The model under review builds one solid part; all positions refer to its coordinate system, in mm. Coordinates: 2 decimals unless noted, no trailing zeros. Loops run counter-clockwise (first coordinate to the right, second up) from the corner with the lowest first, then second, coordinate; pieces in that order, holes last. Notation, with made-up numbers: (76, 67.5) - (90, 67.5) arc R17 cw to (90, 96.5) - close; hole circle Ø5 at (75, 42). An arc over 180 degrees is marked (long way). Answer in a Markdown table with one row per item. Add a question column.
(1) We need section C-C on y = -3. Write out the cut boundary in (x, z).
(2) For P1, Ø4.5, axis at x = -5, y = 0, coming from the -Z side, flat-tipped, find the tip position at first contact; note if it passes through.
(3) We need section A-A on x = 15. Write out the cut boundary in (y, z).
(4) We need section B-B on z = 0.1. Give the number of separate pieces and of enclosed holes in the cut face, plus the area to 3 significant figures.
(5) For line 1 along Y through (x, z) = (-35, 0.25); line 2 along Y through (x, z) = (-26, 0.2); line 3 along X through (y, z) = (2.75, 0.2), list the stretches that pass through material, from the lowest coordinate up.
(6) Mouldability with a two-part tool opening along X and no side actions: class faces 1 (the flat face through (-1, 0, 0.5)), 2 (the cylindrical face through (-3.002, 0.088, 0.246)), 3 (the cylindrical face through (33.153, -0.766, 0.246)), 4 (the cylindrical face through (-50, -0.1, 0.2)) as +X half, -X half, draft (parallel to the pull), parting line (faces both ways), or undercut.
Autodesk Inventor part; units mm, degrees
ref_plane "YZ Plane" through (0, 0, 0) normal (1, 0, 0) x (0, 1, 0)
ref_plane "XZ Plane" through (0, 0, 0) normal (0, 1, 0) x (-1, 0, 0)
ref_plane "XY Plane" through (0, 0, 0) normal (0, 0, 1) x (1, 0, 0)
sketch "Náčrt1" plane through (0, 0, 0) normal (0, 0, 1) x (1, 0, 0)
  line L0 (-45, 0) -> (45, 0) construction
  line L1 (-45, -5) -> (45, -5)
  line L2 (45, 5) -> (-45, 5)
  arc A0 (-45, 5) -> (-45, -5) centre (-45, 0) ccw
  arc A1 (45, -5) -> (45, 5) centre (45, 0) ccw
  point P0 (0, 0)
  point P1 (50, 0)
  dimension "d0" = 50
  dimension "d1" = 5
extrude "Vysunutí1" add sketch "Náčrt1" along normal blind 0.5
sketch "Náčrt2" plane through (0, 0, 0) normal (0, 0, -1) x (-1, 0, 0)
  arc A0 (45, -5) -> (45, 5) centre (45, 0) ccw
  circle A1 centre (45, 0) radius 2
  point P0 (0, 0)
  dimension "d4" = 4
extrude "Vysunutí2" cut sketch "Náčrt2" against normal through all
pattern_linear "Obdélníkové pole1" count 10 spacing 10 along (1, 0, 0) of "Vysunutí2"
properties part number "1010"
Outcome:
| question | item | result |
|---|---|---|
| 1 | outline | (-49, 0) - (49, 0) - (49, 0.5) - (-49, 0.5) - close |
| 2 | P1 | z = 0 |
| 3 | outline | (-5, 0) - (-2, 0) - (-2, 0.5) - (-5, 0.5) - close; (2, 0) - (5, 0) - (5, 0.5) - (2, 0.5) - close |
| 4 | separate pieces | 1 |
| 4 | enclosed holes | 10 |
| 4 | area | 853 mm² |
| 5 | line 1 | -5 to -2, 2 to 5 |
| 5 | line 2 | -5 to -1.73, 1.73 to 5 |
| 5 | line 3 | -49.18 to 49.18 |
| 6 | face 1 | draft |
| 6 | face 2 | undercut |
| 6 | face 3 | undercut |
| 6 | face 4 | -X half |
